Autodesk Fusion 360 part; units mm, degrees
sketch "Sketch1" plane through (0, 0, 0) normal (0, 0, 1) x (1, 0, 0)
  circle A0 centre (0, 0) radius 17
  circle A1 centre (0, 0) radius 25
  dimension "d1" = 34
  dimension "d2" = 50
ref_plane "WorkPlane1" through (0, 0, 12) normal (0, 0, 1) x (1, 0, 0)
sketch "Sketch2" plane through (0, 0, 12) normal (0, 0, 1) x (1, 0, 0)
  circle A0 centre (0, 0) radius 32.5
  dimension "d4" = 65
loft "Loft1" add profiles "Sketch2", "Sketch1" section 1 section 2
extrude "Extrude1" add sketch "Sketch1" against normal blind 6.5
fillet "Fillet1" radius 1.5 1 edges at (-30.3006, 11.7525, 12)
fillet "Fillet2" radius 20 1 edges at (-23.3082, -9.0404, 0)
fillet "Fillet3" radius 5 1 edges at (-23.3082, 9.0404, -6.5)
sketch "Sketch3" plane through (0, 0, 12) normal (0, 0, 1) x (-1, 0, 0)
  circle A0 centre (0, 0) radius 29.7936
  circle A1 centre (0, 0) radius 25
  dimension "d13" = 50
extrude "Extrude2" cut sketch "Sketch3" against normal blind 7.5 contours A1
fillet "Fillet4" radius 2.5 1 edges at (23.3082, -9.0404, 4.5)
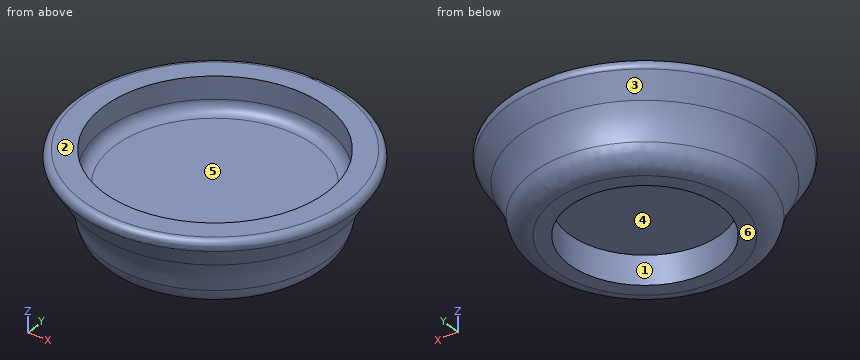
Geometry: final body of the model. Coordinates: model frame, mm. Face numbers are marked on the shaded views. A direction names the side the tool comes from. Round coordinates to 2 decimals unless told otherwise and drop trailing zeros. Write each question's results on one line, items separated by ' | '.
Q1. Pull-direction query (X, two-part tool) for the marked faces 1, 2 and 3; classes: released by +X, released by -X, zero draft, split by the parting line, or undercut.
Response values:
face 1: undercut | face 2: zero draft | face 3: split by the parting line
Q2. Ray query, line 1 along Z through (x, y) = (3, -15); line 2 along X through (y, z) = (1.5, -3.25); line 3 along X through (y, z) = (-12.5, 7.5). Return the intervals inside material, ascending.
Response values:
line 1: 0 to 4.5 | line 2: -25 to -16.93, 16.93 to 25 | line 3: -26.93 to -21.65, 21.65 to 26.93
Q3. Pin query (flat end, axial travel): pin 1 Ø1 at (x, z) = (21.5, 1.5) entering from -Y; pin 2 Ø1.5 at (y, z) = (-21.5, 7) entering from -X; pin 3 Ø4 at (x, y) = (-4, 10) entering from +Z. Return the tip coordinate at first contact, or that it passes through.
Response values:
pin 1: y = -16 | pin 2: x = -21.04 | pin 3: z = 4.5
Q4. Access query for the marked faces 4, 5 and 6. Directions: +Z, -Z, +X, -X, +Y, -Y. A direction counts if a zero-diameter tool reaches every point of the face in a straight line with its end or side. Return the directions, or none.
Response values:
face 4: -Z | face 5: +Z | face 6: -Z, +X, -X, +Y, -Y
